from build123d import *

# Parameters (mm, degrees)
F0_R     = 21.5
F0_R_2   = 20
F1_DEPTH = 22
F2_R     = 22.5
F3_DEPTH = 3
F4_R     = 2.5
F5_DEPTH = 3


with BuildPart() as f1:
    # F0 (on Front) → F1 (new body)
    with BuildSketch(Plane.XZ):
        Circle(F0_R)
        Circle(F0_R_2, mode=Mode.SUBTRACT)
    extrude(amount=F1_DEPTH)

    # F2 (on face) → F3 (join)
    with BuildSketch(Plane.XZ.offset(22)):
        Circle(F2_R)
    extrude(amount=F3_DEPTH)

    # F4 (on face) → F5 (cut)
    with BuildSketch(Plane.XZ.offset(25)):
        Circle(F4_R)
    extrude(amount=-F5_DEPTH, mode=Mode.SUBTRACT)


solid = f1.part
Source: CAD feature listing. Evaluate the final solid. Frame: model axes, mm. A direction names the side the tool comes from. Coordinates: 2 decimals unless noted, no trailing zeros. Loops run counter-clockwise (first coordinate to the right, second up) from the corner with the lowest first, then second, coordinate; pieces in that order, holes last. Notation, with made-up numbers: M -22,42.25 L -1,42.25 A21 cw -1,63.25 Z; hole C -5,73 d3. An arc over 180 degrees is marked long. Answer in a Markdown table with one row per item.
Q1. Section B-B on z = 0. Return the cut outline in (x, y), plus the area to 3 significant figures.
Answers below:
| item | result |
|---|---|
| outline | M -22.5,-25 L -2.5,-25 L -2.5,-22 L -20,-22 L -20,0 L -21.5,0 L -21.5,-22 L -22.5,-22 Z; M 2.5,-25 L 22.5,-25 L 22.5,-22 L 21.5,-22 L 21.5,0 L 20,0 L 20,-22 L 2.5,-22 Z |
| area | 186 mm^2 |
Q2. Section D-D on z = 14. Return the cut outline in (x, y).
Answers below:
| item | result |
|---|---|
| outline | M -17.61,-25 L 17.61,-25 L 17.61,-22 L 16.32,-22 L 16.32,0 L 14.28,0 L 14.28,-22 L -14.28,-22 L -14.28,0 L -16.32,0 L -16.32,-22 L -17.61,-22 Z |
Q3. First-contact query: pin 1 (12 mm diameter, centred on x = -1, y = -17, fed in from +Z); pin 2 (6 mm diameter, centred on x = 12.5, y = -6.5, fed in from +Z); pin 3 (10 mm diameter, centred on x = 11.5, y = -12, fed in from +Z). Flat tips, straight axial feed; report the tip coordinate or a pass-through.
Answers below:
| item | result |
|---|---|
| pin 1 | stops at z = 22.5 |
| pin 2 | stops at z = 19.29 |
| pin 3 | stops at z = 20.49 |
Q4. Ray query, probe 1 along Z at (x, y) = (0, -10); probe 2 along Z at (x, y) = (0, -22.7); probe 3 along Y at (x, z) = (-10.5, 1.5). Return the intervals inside material, ascending. Write a range as from..to.
Answers below:
| item | result |
|---|---|
| probe 1 | z = -21.5..-20, 20..21.5 |
| probe 2 | z = -22.5..-2.5, 2.5..22.5 |
| probe 3 | y = -25..-22 |
Q5. Set-up query: faces 1 (the cylindrical face through (-0.54, -23.52, -2.44)), 2 (the flat face through (22, -22, -2)). Return all of +Z, -Z, +X, -X, +Y, -Y with unobstructed straight access to the full face (end or side cutting, diameter ignored); none if empty.
Answers below:
| item | result |
|---|---|
| face 1 | +Y, -Y |
| face 2 | +Y |
Q6. Section A-A on x = 0. Return the cut outline in (y, z), plus the area to 3 significant figures.
Answers below:
| item | result |
|---|---|
| outline | M -25,-22.5 L -22,-22.5 L -22,-21.5 L 0,-21.5 L 0,-20 L -22,-20 L -22,-2.5 L -25,-2.5 Z; M -25,2.5 L -22,2.5 L -22,20 L 0,20 L 0,21.5 L -22,21.5 L -22,22.5 L -25,22.5 Z |
| area | 186 mm^2 |
Q7. Draft query along Z for faces 3 (the cylindrical face through (10.382, -23.479, -19.961)), 4 (the flat face through (16, 0, -13)), 5 (the cylindrical face through (-4.336, -10.846, -19.524)). Return one class per face: pulls with the +Z half, pulls with the -Z half, needs draft (parallel to the pull), parting line crosses it, or undercut.
Answers below:
| item | result |
|---|---|
| face 3 | parting line crosses it |
| face 4 | needs draft |
| face 5 | undercut |
Q8. Section C-C on x = -12.5. Return the cut outline in (y, z).
Answers below:
| item | result |
|---|---|
| outline | M -25,-18.71 L -22,-18.71 L -22,-17.49 L 0,-17.49 L 0,-15.61 L -22,-15.61 L -22,15.61 L 0,15.61 L 0,17.49 L -22,17.49 L -22,18.71 L -25,18.71 Z |
